Autodesk Inventor part; units mm, degrees
ref_plane "YZ Plane" through (0, 0, 0) normal (1, 0, 0) x (0, 1, 0)
ref_plane "XZ Plane" through (0, 0, 0) normal (0, 1, 0) x (-1, 0, 0)
ref_plane "XY Plane" through (0, 0, 0) normal (0, 0, 1) x (1, 0, 0)
sketch "Sketch1" plane through (0, 0, 0) normal (0, 1, 0) x (-1, 0, 0)
  line L0 (-167.3432, 71.9578) -> (-167.3432, -77.8672)
  line L1 (-162.3432, 76.9578) -> (-0.8632, 76.9578)
  line L2 (11.7368, 76.9578) -> (173.2198, 76.9578)
  arc A0 (-162.3432, 76.9578) -> (-167.3432, 71.9578) centre (-162.3432, 71.9578) ccw
  arc A1 (-167.3432, -77.8672) -> (-162.3432, -82.8672) centre (-162.3432, -77.8672) ccw
  line L3 (178.2198, -77.8672) -> (178.2198, 71.9578)
  line L4 (173.2198, -82.8672) -> (-162.3432, -82.8672)
  arc A2 (173.2198, -82.8672) -> (178.2198, -77.8672) centre (173.2198, -77.8672) ccw
  arc A3 (178.2198, 71.9578) -> (173.2198, 76.9578) centre (173.2198, 71.9578) ccw
  line L5 (-149.3552, 61.9583) -> (1.1368, 61.9583)
  line L6 (9.7368, 61.9583) -> (160.2077, 61.9583)
  line L7 (-152.3432, 58.9581) -> (-152.3432, -64.8672)
  line L8 (163.2197, 58.9581) -> (163.2197, -64.8672)
  line L9 (-149.3432, -67.8672) -> (160.2197, -67.8672)
  arc A4 (-149.3432, 61.9583) -> (-152.3432, 58.9289) centre (-149.3432, 58.9581) ccw
  arc A5 (163.2197, 58.9581) -> (160.2077, 61.9583) centre (160.3139, 59.0529) ccw
  arc A6 (160.2197, -67.8672) -> (163.2197, -64.8672) centre (160.2197, -64.8672) ccw
  arc A7 (-152.3432, -64.8672) -> (-149.3432, -67.8672) centre (-149.3432, -64.8672) ccw
  line L10 (1.1368, 72.9578) -> (1.1368, 61.9583)
  line L11 (9.7368, 72.9578) -> (9.7368, 61.9583)
  line L12 (1.1368, 72.9578) -> (-0.8632, 72.9578)
  line L13 (9.7368, 72.9578) -> (11.7368, 72.9578)
  line L14 (11.7368, 72.9578) -> (11.7368, 76.9578)
  line L15 (-0.8632, 72.9578) -> (-0.8632, 76.9578)
  point P0 (0, 0)
extrude "Extrusion1" add sketch "Sketch1" along normal blind 4
properties part number "layer4"
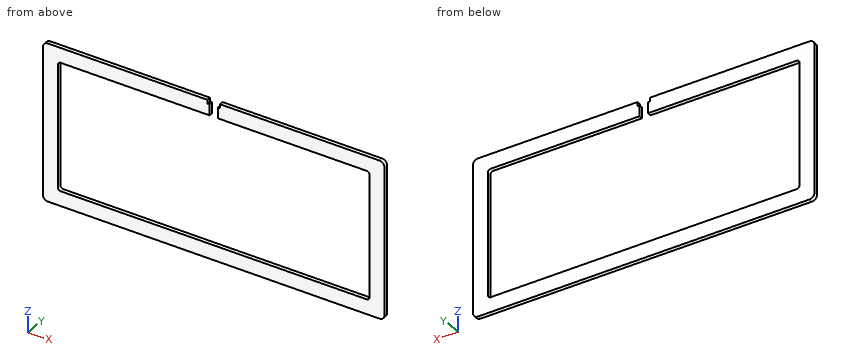
Work out the finished part from the listing and answer in its coordinate system (mm). Round coordinates to 2 decimals unless told otherwise and drop trailing zeros. Loops run counter-clockwise (first coordinate to the right, second up) from the corner with the lowest first, then second, coordinate; pieces in that order, holes last. Notation, with made-up numbers: (58, -35) - (99, -35) arc R20 ccw to (99, -12) - close; hole circle Ø1 at (68, 42.25). An arc over 180 degrees is marked (long way). One line per item, written item: value.
Q1. Find section A-A on x = 83.5. Give the vertices of the cut face in (y, z).
Check values:
outline: (0, -82.87) - (4, -82.87) - (4, -67.87) - (0, -67.87) - close; (0, 61.96) - (4, 61.96) - (4, 76.96) - (0, 76.96) - close
Q2. Each of these flat-tipped pins is pushed along its axis until it touches: pin 1 Ø2 at (x, y) = (-0.5, 2) entering from +Z; pin 2 Ø10 at (x, z) = (-66, -61.5) entering from +Y; pin 3 Ø1.2 at (y, z) = (2, 74.5) entering from +X; pin 4 Ø1.2 at (y, z) = (1, 75.5) entering from -X. Where does it stop, or does it pass through?
Check values:
pin 1: z = 72.96
pin 2: through
pin 3: x = 166.95
pin 4: x = -177.26
Q3. Find section C-C on y = 2.35. Give the vertices of the cut face in (x, z).
Check values:
outline: (-178.22, -77.87) arc R5 ccw to (-173.22, -82.87) - (162.34, -82.87) arc R5 ccw to (167.34, -77.87) - (167.34, 71.96) arc R5 ccw to (162.34, 76.96) - (0.86, 76.96) - (0.86, 72.96) - (-1.14, 72.96) - (-1.14, 61.96) - (149.36, 61.96) arc R3 cw to (152.34, 58.96) - (152.34, -64.87) arc R3 cw to (149.34, -67.87) - (-160.22, -67.87) arc R3 cw to (-163.22, -64.87) - (-163.22, 58.96) arc R2.91 cw to (-160.21, 61.96) - (-9.74, 61.96) - (-9.74, 72.96) - (-11.74, 72.96) - (-11.74, 76.96) - (-173.22, 76.96) arc R5 ccw to (-178.22, 71.96) - close
Q4. Straight lines are drawn through the part: probe 1 along Z at (x, y) = (-134, 1.15); probe 2 along X at (y, z) = (3.05, -31); probe 3 along Z at (x, y) = (-7, 1.45). For each, find the intervals that lie inside material, in ascending order.
Check values:
probe 1: -82.87 to -67.87, 61.96 to 76.96
probe 2: -178.22 to -163.22, 152.34 to 167.34
probe 3: -82.87 to -67.87
Q5. Find section B-B on z = 14.5. Give the vertices of the cut face in (x, y), and give its area (3 significant figures).
Check values:
outline: (-178.22, 0) - (-163.22, 0) - (-163.22, 4) - (-178.22, 4) - close; (152.34, 0) - (167.34, 0) - (167.34, 4) - (152.34, 4) - close
area: 120 mm2
